```python
from build123d import *

# Parameters (mm, degrees)
SKETCH_1_R               = 17
EXTRUDE_1_DEPTH          = 4
EXTRUDE_2_DEPTH          = 1
FILLET_1_R               = 1.55
FILLET_2_R               = 0.8
SKETCH_3_R               = 6.5
CUT_EXTRUDE_1_DEPTH      = 6
SKETCH_4_R               = 1.25
CUT_EXTRUDE_2_DEPTH      = 6.0000001
PATTERN_CIRCULAR_1_COUNT = 2
PATTERN_CIRCULAR_1_ANGLE = 45


with BuildPart() as part:
    # ｽｹｯﾁ1 → ﾎﾞｽ - 押し出し1 (new body)
    with BuildSketch(Plane.XY):
        Circle(SKETCH_1_R)
    extrude(amount=EXTRUDE_1_DEPTH)

    # ｽｹｯﾁ2 → ﾎﾞｽ - 押し出し2 (add)
    with BuildSketch(Plane.XY.offset(4)):
        with BuildLine():
            Line((-1.5, 14.422205102), (-1.5, 12.5))
            Line((-1.5, 12.5), (1.5, 12.5))
            Line((1.5, 12.5), (1.5, 14.422205102))
            ThreePointArc((1.5, 14.422205102), (0, 14.5), (-1.5, 14.422205102))
        make_face()
        with BuildLine():
            Line((1.5, 12.5), (-1.5, 12.5))
            Line((-1.5, 12.5), (-1.5, 14.422205102))
            ThreePointArc((-1.5, 14.422205102), (-9.708243919, -10.770329614), (14.5, 0))
            ThreePointArc((14.5, 0), (10.770329614, 9.708243919), (1.5, 14.422205102))
            Line((1.5, 14.422205102), (1.5, 12.5))
        make_face()
        with BuildLine():
            Line((-1.5, 16.5), (-1.5, 14.422205102))
            ThreePointArc((-1.5, 14.422205102), (0, 14.5), (1.5, 14.422205102))
            Line((1.5, 14.422205102), (1.5, 16.5))
            Line((1.5, 16.5), (-1.5, 16.5))
        make_face()
    extrude(amount=EXTRUDE_2_DEPTH)

    # ﾌｨﾚｯﾄ1
    fillet_1_edges = [part.edges().sort_by_distance(p)[0] for p in [
        (-1.5, 14.422205102, 4.5),
        (1.5, 14.422205102, 4.5),
    ]]
    fillet(fillet_1_edges, radius=FILLET_1_R)

    # ﾌｨﾚｯﾄ2
    fillet_2_edges = [part.edges().sort_by_distance(p)[0] for p in [
        (1.5, 16.5, 4.5),
        (-1.5, 16.5, 4.5),
    ]]
    fillet(fillet_2_edges, radius=FILLET_2_R)

    # ｽｹｯﾁ3 → ｶｯﾄ - 押し出し1 (cut, through all)
    with BuildSketch(Plane.XY.offset(5)):
        Circle(SKETCH_3_R)
    extrude(amount=-CUT_EXTRUDE_1_DEPTH, mode=Mode.SUBTRACT)

    # ｽｹｯﾁ4 → ｶｯﾄ - 押し出し2 (cut, through all)
    with BuildSketch(Plane(origin=(0, 0, 0), x_dir=(-1, 0, 0), z_dir=(0, 0, -1))):
        with Locations((0, 12)):
            Circle(SKETCH_4_R)
        with Locations((12, 0)):
            Circle(SKETCH_4_R)
        with Locations((0, -12)):
            Circle(SKETCH_4_R)
        with Locations((-12, 0)):
            Circle(SKETCH_4_R)
    cut_extrude_2 = extrude(amount=-CUT_EXTRUDE_2_DEPTH, mode=Mode.SUBTRACT)

    # 円形ﾊﾟﾀｰﾝ1: ｶｯﾄ - 押し出し2 ×2 about axis
    pattern_circular_1_axis = Axis((0, 0, 0), (0, 0, 1))
    for i in range(1, PATTERN_CIRCULAR_1_COUNT):
        add(cut_extrude_2.rotate(pattern_circular_1_axis, i * PATTERN_CIRCULAR_1_ANGLE / (PATTERN_CIRCULAR_1_COUNT - 1)), mode=Mode.SUBTRACT)


solid = part.part
```
CAD build for the part. Positions are in the model's coordinates, mm. A direction names the side the tool comes from. Coordinates: 2 decimals unless noted, no trailing zeros. Order: outer loops, then holes, each group sorted by start corner. A loop starts at its lowest first (then second) coordinate and runs counter-clockwise, first axis right, second up. Notation, with made-up numbers: M 0,29.5 L 14,29.5 A24 ccw 14,49.5 Z; hole C 14.5,-22 d8. An arc over 180 degrees is marked long. Write each question's results on one line, items separated by ' | '. Start each with the question number.
Q1. Cut at D-D (z = 0.8). Count the separate pieces of the cut face and the enclosed holes in it, then the cut area to 3 significant figures.
Q2. Cut at C-C (x = -6). List the corners of the cut face in (y, z), then the cut area to 3 significant figures.
Q3. Cut at B-B (y = -12). List the corners of the cut face in (x, z), then the cut area to 3 significant figures.
Q4. Drill centre lines: probe 1 along Y at (x, z) = (0, 2.6); probe 2 along X at (y, z) = (1, 1.5); probe 3 along Y at (x, z) = (-9.5, 0.8). Where is each one in solid material? Low to high. Write a range as from..to.
Q5. Cut at A-A (x = 0). List the corners of the cut face in (y, z), then the cut area to 3 significant figures.
Q6. Flat gauge pins, fed straight in: P1, Ø2, axis at y = -7.5, z = 2.5, coming from the +X side; P2, Ø1, axis at x = -10.5, z = 2, coming from the -Y side. Where does each tip first touch, or does it go through?
Q7. Pull direction X, two halves, no side cores. Call faces 3 (the cylindrical face through (-1.876, 14.745, 4.507)), 4 (the cylindrical face through (-9.706, 8.755, 2.465)), 5 (the cylindrical face through (1.876, 14.745, 4.507)), 6 (the flat face through (0, 16.5, 4.5)): +X half, -X half, draft (parallel to the pull), parting line (faces both ways), or undercut.
Q8. Which spindle directions (+Z, -Z, +X, -X, +Y, -Y) get a long thin tool onto all of the face, cutting with end or side? Do faces 1 (the flat face through (7, -13, 4)), 2 (the cylindrical face through (-10.75, 0.05, 2.46)). Say none if no direction does.
Found:
1) separate pieces: 1 | enclosed holes: 9 | area: 736 mm²
2) outline: M -15.91,0 L -2.5,0 L -2.5,5 L -13.2,5 L -13.2,4 L -15.91,4 Z; M 2.5,0 L 15.91,0 L 15.91,4 L 13.2,4 L 13.2,5 L 2.5,5 Z | area: 129 mm²
3) outline: M -12.04,0 L -1.25,0 L -1.25,5 L -8.14,5 L -8.14,4 L -12.04,4 Z; M 1.25,0 L 12.04,0 L 12.04,4 L 8.14,4 L 8.14,5 L 1.25,5 Z | area: 100 mm²
4) probe 1: -17..-13.25, -10.75..-6.5, 6.5..10.75, 13.25..17 | probe 2: -16.97..-12.75, -11.25..-6.42, 6.42..11.25, 12.75..16.97 | probe 3: -14.1..-9.22, -7.76..7.76, 9.22..14.1
5) outline: M -17,0 L -13.25,0 L -13.25,5 L -14.5,5 L -14.5,4 L -17,4 Z; M -10.75,0 L -6.5,0 L -6.5,5 L -10.75,5 Z; M 6.5,0 L 10.75,0 L 10.75,5 L 6.5,5 Z; M 13.25,0 L 17,0 L 17,4 L 16.5,4 L 16.5,5 L 13.25,5 Z | area: 77.0 mm²
6) P1: x = 15.71 | P2: y = -13.75
7) face 3: -X half | face 4: undercut | face 5: +X half | face 6: draft
8) face 1: +Z | face 2: +Z, -Z
